from build123d import *

# Parameters (mm, degrees)
SKETCH_1_W = 1.5
SKETCH_1_H = 2.5
FILLET_1_R = 0.3


with BuildPart() as part:
    # Эскиз1 → Повернуть1 (revolve)
    with BuildSketch(Plane.XY, mode=Mode.PRIVATE) as revolve_1_sk:
        with Locations((-8.75, 1.25)):
            Rectangle(SKETCH_1_W, SKETCH_1_H)
    revolve(revolve_1_sk.sketch.rotate(Axis((0, 0, 0), (0, 1, 0)), 270), axis=Axis((0, 0, 0), (0, 1, 0)))

    # Скругление1
    fillet_1_edges = [part.edges().sort_by_distance(p)[0] for p in [
        (0, 2.5, 9.5),
        (0, 2.5, 8),
        (0, 0, 8),
        (0, 0, 9.5),
    ]]
    fillet(fillet_1_edges, radius=FILLET_1_R)


solid = part.part
The model under review builds one solid part; all positions refer to its coordinate system, in mm. Round coordinates to 2 decimals unless told otherwise and drop trailing zeros. Loops run counter-clockwise (first coordinate to the right, second up) from the corner with the lowest first, then second, coordinate; pieces in that order, holes last. Notation, with made-up numbers: M 45.5,46 L 53.5,46 A19 ccw 53.5,79 Z; hole C 81.25,55 d4. An arc over 180 degrees is marked long. Answer as a JSON object with one key per item and string values.
Item 1: We need section B-B, the plane z = 0. State the section outline as (x, y) points.
Check sheet entries:
{"outline": "M -9.5,0.3 A0.3 ccw -9.2,0 L -8.3,0 A0.3 ccw -8,0.3 L -8,2.2 A0.3 ccw -8.3,2.5 L -9.2,2.5 A0.3 ccw -9.5,2.2 Z; M 8,0.3 A0.3 ccw 8.3,0 L 9.2,0 A0.3 ccw 9.5,0.3 L 9.5,2.2 A0.3 ccw 9.2,2.5 L 8.3,2.5 A0.3 ccw 8,2.2 Z"}
Item 2: We need section C-C, the plane y = 0.9. State the section outline as (x, z) points.
Check sheet entries:
{"outline": "C 0,0 d19; hole C 0,0 d16"}
Item 3: The part is to be moulded in two halves that separate along X. For faces 1 (the face through (-7, 0, 5)), 2 (the face through (7.81, 1.26, 1.73)), 3 (the face through (5.78, 1.26, 7.54)), say which applies: +X half, -X half, draft (parallel to the pull), parting line (faces both ways), or undercut.
Check sheet entries:
{"face 1": "draft", "face 2": "undercut", "face 3": "parting line"}
Item 4: For line 1 along X through (y, z) = (1.6, 0); line 2 along Z through (x, y) = (-3.5, 2.1); line 3 along Z through (x, y) = (-7, 1.85), list the stretches that pass through material, from the lowest coordinate up.
Check sheet entries:
{"line 1": "-9.5 to -8, 8 to 9.5", "line 2": "-8.83 to -7.19, 7.19 to 8.83", "line 3": "-6.42 to -3.87, 3.87 to 6.42"}
Item 5: We need section A-A, the plane x = 0. State the section outline as (y, z) points.
Check sheet entries:
{"outline": "M 0,-9.2 A0.3 ccw 0.3,-9.5 L 2.2,-9.5 A0.3 ccw 2.5,-9.2 L 2.5,-8.3 A0.3 ccw 2.2,-8 L 0.3,-8 A0.3 ccw 0,-8.3 Z; M 0,8.3 A0.3 ccw 0.3,8 L 2.2,8 A0.3 ccw 2.5,8.3 L 2.5,9.2 A0.3 ccw 2.2,9.5 L 0.3,9.5 A0.3 ccw 0,9.2 Z"}
